Geometry check sheet. Reference: the model listing, model coordinates, mm. Round coordinates to 2 decimals unless told otherwise and drop trailing zeros. Write each loop counter-clockwise with the first axis right and the second up, starting at its lowest first coordinate (ties: lowest second). Pieces come first, ordered by that corner, then holes.
Item 1: Depth check by flat-ended pin: P1, Ø2, axis at y = 24.5, z = 22, coming from the +X side; P2, Ø1, axis at x = 12.5, y = 11.5, coming from the -Z side; P3, Ø8, axis at y = 17.5, z = 15.5, coming from the -X side. Enter the tip coordinate at first touch or a pass-through.
Item 2: Draft check along X on faces 1 (the face through (-15.02, 16.18, -47.69)), 2 (the face through (0.676, 27.707, 2.146)), 3 (the face through (-1, 0, -1)). Enter one of: pulls with the +X half, pulls with the -X half, needs draft (parallel to the pull), parting line crosses it, or undercut.
Item 3: Scan lines: probe 1 along X at (y, z) = (30, -5.5); probe 2 along X at (y, z) = (30, 3.5); probe 3 along X at (y, z) = (29, 0). Record each from-to range of solid material in increasing order.
Item 4: Cross-section at A-A (y = 5.5). Enter the section's corners in (x, z), then the cut area to 3 significant figures.
from build123d import *

# Parameters (mm, degrees)
FILLET1_R          = 3
SKETCH2_R          = 2.25
CUT_EXTRUDE1_DEPTH = 30


with BuildPart() as part:
    # Sketch1 → Revolve1 (revolve)
    with BuildSketch(Plane.XY, mode=Mode.PRIVATE) as revolve1_sk:
        with BuildLine():
            Line((0, 0), (50, 0))
            Line((50, 0), (50, 35))
            add(Edge.make_bspline(
                [(0, 35), (20.190635026, 38.073649128), (11.656369597, 5.024124106), (50, 35)],
                knots=[0, 0, 0, 0, 1, 1, 1, 1], degree=3))
            Line((0, 35), (0, 0))
        make_face()
    revolve(revolve1_sk.sketch.rotate(Axis((0, 0, 0), (0, 1, 0)), 90), axis=Axis((0, 0, 0), (0, 1, 0)))

    # Fillet1
    fillet1_edges = [part.edges().sort_by_distance(p)[0] for p in [
        (0, 35, 50),
        (0, 0, 50),
    ]]
    fillet(fillet1_edges, radius=FILLET1_R)

    # Sketch2 → Cut-Extrude1 (cut)
    with BuildSketch(Plane(origin=(0, 50, 0), x_dir=(1, 0, 0), z_dir=(0, 1, 0))):
        with Locations(Location((0, 0, 0), (0, 0, 270))):
            Circle(SKETCH2_R)
    extrude(amount=-CUT_EXTRUDE1_DEPTH, mode=Mode.SUBTRACT)


solid = part.part
Resolved:
1. P1: stops at x = 45.38
1. P2: stops at z = -48.54
1. P3: stops at x = -48.66
2. face 1: parting line crosses it
2. face 2: undercut
2. face 3: needs draft
3. probe 1: x = -49.52 to -42.85, -11.93 to 11.93, 42.85 to 49.52
3. probe 2: x = -49.7 to -43.06, -12.66 to 12.66, 43.06 to 49.7
3. probe 3: x = -50 to -41.71, -14.07 to -2.25, 2.25 to 14.07, 41.71 to 50
4. outline: circle Ø100 at (0, 0)
4. area: 7,850 mm2
